Input: part model. Units: mm. Frame: model coordinates. A direction names the side the tool comes from. Give positions to 0.01 mm unless a question says otherwise; leave off trailing zeros. Loops run counter-clockwise (first coordinate to the right, second up) from the corner with the lowest first, then second, coordinate; pieces in that order, holes last.
from build123d import *

# Parameters (mm, degrees)
SKETCH1_R           = 6.5
BOSS_EXTRUDE1_DEPTH = 2.5
SKETCH2_R           = 4.75
SKETCH2_R_2         = 3
BOSS_EXTRUDE2_DEPTH = 13
SKETCH3_W           = 8
SKETCH3_H           = 7
BOSS_EXTRUDE3_DEPTH = 11.5
FILLET1_R           = 4
SKETCH4_R           = 1.5
CUT_EXTRUDE1_DEPTH  = 13
SKETCH5_W           = 3
SKETCH5_H           = 10.207029109
CUT_EXTRUDE2_DEPTH  = 13


with BuildPart() as part:
    # Sketch1 → Boss-Extrude1 (new body)
    with BuildSketch(Plane(origin=(0, 0, 0), x_dir=(1, 0, 0), z_dir=(0, 1, 0))):
        with Locations(Location((0, 0, 0), (0, 0, 270))):
            Circle(SKETCH1_R)
    extrude(amount=BOSS_EXTRUDE1_DEPTH)

    # Sketch2 → Boss-Extrude2 (add)
    with BuildSketch(Plane.XZ):
        with Locations(Location((0, 0, 0), (0, 0, 90))):
            Circle(SKETCH2_R)
        with Locations(Location((0, 0, 0), (0, 0, 90))):
            Circle(SKETCH2_R_2, mode=Mode.SUBTRACT)
    extrude(amount=BOSS_EXTRUDE2_DEPTH)

    # Sketch3 → Boss-Extrude3 (add)
    with BuildSketch(Plane(origin=(0, 2.5, 0), x_dir=(1, 0, 0), z_dir=(0, 1, 0))):
        Rectangle(SKETCH3_W, SKETCH3_H)
    extrude(amount=BOSS_EXTRUDE3_DEPTH)

    # Fillet1
    fillet1_edges = [part.edges().sort_by_distance(p)[0] for p in [
        (4, 14, 0),
        (-4, 14, 0),
    ]]
    fillet(fillet1_edges, radius=FILLET1_R - 0.0001)  # a hair under: the kernel refuses the full size

    # Sketch4 → Cut-Extrude1 (cut)
    with BuildSketch(Plane.XY.offset(3.5)):
        with Locations((0, 10)):
            Circle(SKETCH4_R)
    extrude(amount=-CUT_EXTRUDE1_DEPTH, mode=Mode.SUBTRACT)

    # Sketch5 → Cut-Extrude2 (cut)
    with BuildSketch(Plane.ZY.offset(4)):
        with Locations((0, 13.103514555)):
            Rectangle(SKETCH5_W, SKETCH5_H)
    extrude(amount=-CUT_EXTRUDE2_DEPTH, mode=Mode.SUBTRACT)


solid = part.part
(1) Mould query, pull axis X, two halves, no side actions, for faces 6 (the cylindrical face through (-0.325, 8.536, 2.514)), 7 (the flat face through (0, 12, -1.5)), 8 (the cylindrical face through (2.859, 12.797, 2.486)). Classes: +X half, -X half, draft (parallel to the pull), parting line (faces both ways), or undercut.
Values follow:
face 6: undercut
face 7: draft
face 8: +X half
(2) Ray query, probe 1 along Y at (x, z) = (0, -1.9); probe 2 along Z at (x, y) = (2, 12.5); probe 3 along Y at (x, z) = (1.25, -5.25). Return the intervals inside material, ascending.
Values follow:
probe 1: y = 0 to 8.5, 11.5 to 14
probe 2: z = -3.5 to -1.5, 1.5 to 3.5
probe 3: y = 0 to 2.5
(3) Reachability of faces 1 (the flat face through (0, 8, 0)), 2 (the flat face through (0, 8, -3.5)), 3 (the flat face through (-5, 0, 0)), 4 (the flat face through (-4.2, 2.5, -0.1)), 5 (the flat face through (4, 6, 0)) from +Z, -Z, +X, -X, +Y, -Y: full face, straight path, thin tool, end or side. Return the list, or none.
Values follow:
face 1: +X, -X, +Y
face 2: -Z, +X, -X, +Y
face 3: -Y
face 4: +Y
face 5: +Z, -Z, +X, +Y
(4) Pin query (flat end, axial travel): pin 1 Ø2 at (x, y) = (-1.5, 10) entering from -Z; pin 2 Ø0.9 at (x, z) = (1, 0) entering from +Y; pin 3 Ø5 at (x, z) = (4.5, 5) entering from +Y. Return the tip coordinate at first contact, or that it passes through.
Values follow:
pin 1: stops at z = -3.5
pin 2: stops at y = 8
pin 3: stops at y = 13.12
(5) Cut plane A-A (z = 0). Return the cut outline in (x, y), and give its area (3 significant figures).
Values follow:
outline: (-6.5, 0) - (-4.75, 0) - (-4.75, -13) - (-3, -13) - (-3, 0) - (3, 0) - (3, -13) - (4.75, -13) - (4.75, 0) - (6.5, 0) - (6.5, 2.5) - (4, 2.5) - (4, 8) - (-4, 8) - (-4, 2.5) - (-6.5, 2.5) - close
area: 122 mm2
(6) Cut plane B-B (x = -2). Return the cut outline in (y, z), and give its area (3 significant figures).
Values follow:
outline: (-13, -4.31) - (0, -4.31) - (0, -6.18) - (2.5, -6.18) - (2.5, -3.5) - (13.46, -3.5) - (13.46, -1.5) - (8, -1.5) - (8, 1.5) - (13.46, 1.5) - (13.46, 3.5) - (2.5, 3.5) - (2.5, 6.18) - (0, 6.18) - (0, 4.31) - (-13, 4.31) - (-13, 2.24) - (0, 2.24) - (0, -2.24) - (-13, -2.24) - close
area: 145 mm2
(7) Cut plane D-D (y = -9.25). Return the cut outline in (x, z), and give its area (3 significant figures).
Values follow:
outline: circle Ø9.5 at (0, 0); hole circle Ø6 at (0, 0)
area: 42.6 mm2
(8) Cut plane C-C (y = 5.25). Return the cut outline in (x, z).
Values follow:
outline: (-4, -3.5) - (4, -3.5) - (4, 3.5) - (-4, 3.5) - close
